Geometry check sheet. Reference: the model listing, model coordinates, mm. Give positions to 0.01 mm unless a question says otherwise; leave off trailing zeros. Write each loop counter-clockwise with the first axis right and the second up, starting at its lowest first coordinate (ties: lowest second). Pieces come first, ordered by that corner, then holes. Notation, with made-up numbers: (5, 50.5) - (22, 50.5) arc R33 cw to (22, 79.5) - close; hole circle Ø6 at (-33.5, 34). An arc over 180 degrees is marked (long way). One line per question, with ' | ' between items. Start each with the question number.
Q1. Section check A-A on y = 0. Record the boundary of the cut face in (x, z), and give its area (3 significant figures).
Q2. Gauge pin test, flat ends, axial feed: P1, Ø5, axis at y = -3.5, z = 32, coming from the +X side; P2, Ø1, axis at x = 2.5, z = 63, coming from the -Y side; P3, Ø2, axis at y = -5.5, z = 49, coming from the -X side. Record the tip position at first contact, or that the pin passes through.
Q3. Thickness scan on L1, parallel to Y at x = 0, z = 39; L2, parallel to Y at x = -0.75, z = 19; L3, parallel to Z at x = 4.75, y = 4.25. Record the ranges inside material, lowest first. Write a range as [from, to].
Q4. Section check D-D on x = -8. Record the boundary of the cut face in (y, z).
Q5. Section check B-B on x = 0. Record the boundary of the cut face in (y, z).
Q6. Section check C-C on z = 45.5. Record the boundary of the cut face in (x, y), and give its area (3 significant figures).
```python
from build123d import *

# Parameters (mm, degrees)
SKETCH_1_R      = 10.6
SKETCH_1_R_2    = 2.15
SKETCH_1_R_3    = 4.1
EXTRUDE_1_DEPTH = 79
SKETCH_2_R      = 1.45
EXTRUDE_2_DEPTH = 1.6
CHAMFER_1_SIZE  = 0.3


with BuildPart() as part:
    # 草图1 → 凸台-拉伸1 (new body)
    with BuildSketch(Plane.XY):
        Circle(SKETCH_1_R)
        with Locations((0, 7)):
            Circle(SKETCH_1_R_2, mode=Mode.SUBTRACT)
        Circle(SKETCH_1_R_3, mode=Mode.SUBTRACT)
    extrude(amount=EXTRUDE_1_DEPTH)

    # 草图2 → 凸台-拉伸2 (add)
    with BuildSketch(Plane.XY):
        with Locations((-8, 0)):
            Circle(SKETCH_2_R)
        with Locations((8, 0)):
            Circle(SKETCH_2_R)
    extrude(amount=-EXTRUDE_2_DEPTH)

    # 倒角1
    chamfer_1_edges = [part.edges().sort_by_distance(p)[0] for p in [
        (-2.15, 7, 0),
        (-2.15, 7, 79),
    ]]
    chamfer(chamfer_1_edges, length=CHAMFER_1_SIZE)


solid = part.part
```
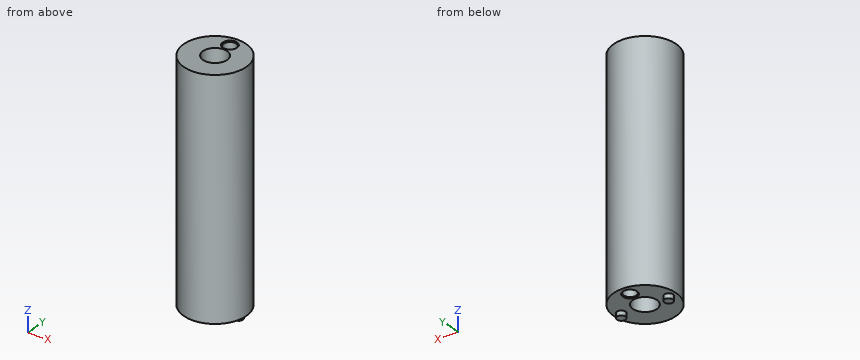
Working result:
1) outline: (-10.6, 0) - (-9.45, 0) - (-9.45, -1.6) - (-6.55, -1.6) - (-6.55, 0) - (-4.1, 0) - (-4.1, 79) - (-10.6, 79) - close; (4.1, 0) - (6.55, 0) - (6.55, -1.6) - (9.45, -1.6) - (9.45, 0) - (10.6, 0) - (10.6, 79) - (4.1, 79) - close | area: 1,040 mm2
2) P1: stops at x = 10.55 | P2: stops at y = -10.41 | P3: stops at x = -9.6
3) L1: y = [-10.6, -4.1], [4.1, 4.85], [9.15, 10.6] | L2: y = [-10.57, -4.03], [4.03, 4.99], [9.01, 10.57] | L3: z = [0, 79]
4) outline: (-6.95, 0) - (-1.45, 0) - (-1.45, -1.6) - (1.45, -1.6) - (1.45, 0) - (6.95, 0) - (6.95, 79) - (-6.95, 79) - close
5) outline: (-10.6, 0) - (-4.1, 0) - (-4.1, 79) - (-10.6, 79) - close; (4.1, 0) - (4.55, 0) - (4.85, 0.3) - (4.85, 78.7) - (4.55, 79) - (4.1, 79) - close; (9.15, 0.3) - (9.45, 0) - (10.6, 0) - (10.6, 79) - (9.45, 79) - (9.15, 78.7) - close
6) outline: circle Ø21.2 at (0, 0); hole circle Ø8.2 at (0, 0); hole circle Ø4.3 at (0, 7) | area: 286 mm2
